Could you check a few things on this model? Use its own coordinates, in mm. A direction names the side the tool comes from. Coordinates: 2 decimals unless noted, no trailing zeros. One line per question, with ' | ' between items.
```python
from build123d import *

# Parameters (mm, degrees)
BOSS_EXTRUDE1_DEPTH = 6
SKETCH2_R           = 5
CUT_EXTRUDE1_DEPTH  = 6
SKETCH11_R          = 4.999999998
CUT_EXTRUDE2_DEPTH  = 10
SKETCH12_R          = 5
SKETCH12_R_2        = 2.5
CUT_EXTRUDE3_DEPTH  = 10
CUT_EXTRUDE4_DEPTH  = 10
CUT_EXTRUDE5_DEPTH  = 10
BOSS_EXTRUDE2_START = -6
SKETCH14_R          = 2.5
BOSS_EXTRUDE2_DEPTH = 6
SKETCH14_3_R        = 2.5
CUT_EXTRUDE6_DEPTH  = 6
SKETCH11_4_R        = 4.999999998
BOSS_EXTRUDE3_DEPTH = 6


with BuildPart() as part:
    # Sketch1 → Boss-Extrude1 (new body)
    with BuildSketch(Plane.XY):
        Polygon((-82.808015356, -91.768584182), (61.688025962, -107.113154668), (120.9333121, 25.569013955), (13.052871288, 122.915674351), (-112.866193993, 50.397050544), align=None)
    extrude(amount=BOSS_EXTRUDE1_DEPTH)

    # Sketch2 → Cut-Extrude1 (cut)
    with BuildSketch(Plane.XY.offset(6)):
        Circle(SKETCH2_R)
    extrude(amount=-CUT_EXTRUDE1_DEPTH, mode=Mode.SUBTRACT)

    # Sketch11 → Cut-Extrude2 (cut)
    with BuildSketch(Plane.XY.offset(6)):
        with Locations((-6.54719671, -61.653339044)):
            Circle(SKETCH11_R)
        with Locations((-4.672797652, -44.002584721)):
            Circle(SKETCH11_R)
        with Locations((-2.798398593, -26.351830398)):
            Circle(SKETCH11_R)
        with Locations((-8.975995491, -84.524739011)):
            Circle(SKETCH11_R)
    cut_extrude2 = extrude(amount=-CUT_EXTRUDE2_DEPTH, mode=Mode.SUBTRACT)

    # Sketch12 → Cut-Extrude3 (cut)
    with BuildSketch(Plane.XY.offset(6)):
        with Locations((48.851207931, -21.813057641)):
            Circle(SKETCH12_R)
        with Locations((25.110433983, -11.212319348)):
            Circle(SKETCH12_R)
        with Locations((84.822429951, -20.352343286)):
            Circle(SKETCH12_R_2)
        with Locations((72.591981879, -32.413795933)):
            Circle(SKETCH12_R)
    cut_extrude3 = extrude(amount=-CUT_EXTRUDE3_DEPTH, mode=Mode.SUBTRACT)

    # Sketch11_3 → Cut-Extrude4 (cut)
    with BuildSketch(Plane.XY.offset(6)):
        Polygon((8.29449613, -101.443097727), (8.875295839, -95.973849909), (23.791426251, -97.557849113), (23.210626543, -103.027096932), align=None)
        Polygon((-29.414485521, -97.438641123), (-28.833685813, -91.969393305), (-43.749816225, -90.3853941), (-44.330615934, -95.854641919), align=None)
    cut_extrude4 = extrude(amount=-CUT_EXTRUDE4_DEPTH, mode=Mode.SUBTRACT)

    # Mirror3: Cut-Extrude2 across plane
    add(cut_extrude2.mirror(Plane(origin=(0, 0, 0), x_dir=(0, 0, 1), z_dir=(-0.4077207035645653, -0.9131066903077734, 0))), mode=Mode.SUBTRACT)

    # Mirror4: Cut-Extrude3 across plane
    add(cut_extrude3.mirror(Plane(origin=(0, 0, 0), x_dir=(0, 0, 1), z_dir=(0.742423441529948, -0.6699309169360882, 0))), mode=Mode.SUBTRACT)

    # Mirror5: Cut-Extrude2 across plane
    add(cut_extrude2.mirror(Plane(origin=(0, 0, 0), x_dir=(0, 0, 1), z_dir=(0.742423441529948, -0.6699309169360882, 0))), mode=Mode.SUBTRACT)

    # Mirror6: Cut-Extrude4 across plane
    add(cut_extrude4.mirror(Plane(origin=(0, 0, 0), x_dir=(0, 0, 1), z_dir=(-0.4077207035645653, -0.9131066903077734, 0))), mode=Mode.SUBTRACT)

    # Mirror7: Cut-Extrude4 across plane
    add(cut_extrude4.mirror(Plane(origin=(0, 0, 0), x_dir=(0, 0, 1), z_dir=(0.742423441529948, -0.6699309169360882, 0))), mode=Mode.SUBTRACT)

    # Sketch13 → Cut-Extrude5 (cut)
    with BuildSketch(Plane.XY.offset(6)):
        Polygon((79.910592339, -66.30299436), (102.710745723, -15.241146353), (97.688658926, -12.998682483), (74.888505542, -64.060530491), align=None)
    cut_extrude5 = extrude(amount=-CUT_EXTRUDE5_DEPTH, mode=Mode.SUBTRACT)

    # Mirror8: Cut-Extrude5 across plane
    add(cut_extrude5.mirror(Plane(origin=(0, 0, 0), x_dir=(0, 0, 1), z_dir=(0.742423441529948, -0.6699309169360882, 0))), mode=Mode.SUBTRACT)

    # Sketch14 → Boss-Extrude2 (add)
    with BuildSketch(Plane(origin=(0, 0, 0), x_dir=(-1, 0, 0), z_dir=(0, 0, -1)).offset(BOSS_EXTRUDE2_START)):
        with Locations((-84.822429951, -20.352343286)):
            Circle(SKETCH14_R)
    extrude(amount=BOSS_EXTRUDE2_DEPTH)

    # Sketch14_3 → Cut-Extrude6 (cut)
    with BuildSketch(Plane(origin=(0, 0, 0), x_dir=(-1, 0, 0), z_dir=(0, 0, -1))):
        with Locations(Location((-71.775367437, -49.571757376, 0), (0, 0, 180))):
            Circle(SKETCH14_3_R)
    extrude(amount=-CUT_EXTRUDE6_DEPTH, mode=Mode.SUBTRACT)

    # Sketch11_4 → Boss-Extrude3 (add)
    with BuildSketch(Plane.XY.offset(6)):
        Polygon((8.875295839, -95.973849909), (8.29449613, -101.443097727), (23.210626543, -103.027096932), (23.791426251, -97.557849113), align=None)
        Polygon((-44.330615934, -95.854641919), (-29.414485521, -97.438641123), (-28.833685813, -91.969393305), (-43.749816225, -90.3853941), align=None)
        with Locations((-6.54719671, -61.653339044)):
            Circle(SKETCH11_4_R)
        with Locations((-4.672797652, -44.002584721)):
            Circle(SKETCH11_4_R)
        with Locations((-2.798398593, -26.351830398)):
            Circle(SKETCH11_4_R)
        with Locations((-8.975995491, -84.524739011)):
            Circle(SKETCH11_4_R)
    extrude(amount=-BOSS_EXTRUDE3_DEPTH)

    # Mirror9: Cut-Extrude3, Cut-Extrude5 across plane
    add(cut_extrude3.mirror(Plane(origin=(0, 0, 0), x_dir=(0, 0, 1), z_dir=(0.8665636244747431, 0.4990666135268884, 0))), mode=Mode.SUBTRACT)
    add(cut_extrude5.mirror(Plane(origin=(0, 0, 0), x_dir=(0, 0, 1), z_dir=(0.8665636244747431, 0.4990666135268884, 0))), mode=Mode.SUBTRACT)


solid = part.part
```
Q1. For faces 1 (the face through (43.742, 87.815, 3.042)), 2 (the face through (-88.084, -53.335, 3.042)), 3 (the face through (70.672, -86.994, 2.958)), 4 (the face through (-38.078, -93.792, 3.042)), which set-ups out of +Z, -Z, +X, -X, +Y, -Y let a thin tool reach every point of the face, with its end or its side?
Values follow:
face 1: +Z, -Z | face 2: +Z, -Z, -X | face 3: +Z, -Z, +X, -Y | face 4: +Z, -Z, -Y
Q2. Imagine slicing it at A-A on z = 5. Give the number of separate pieces and of enclosed holes in the cut face, plus the area to 3 significant figures.
Values follow:
separate pieces: 1 | enclosed holes: 21 | area: 33,600 mm2
Q3. Please list where these lines run through material, in increasing order: L1, parallel to X at y = 84, z = 4.25; L2, parallel to Y at x = 75, z = 3.25; L3, parallel to X at y = -7.5, z = 4.75. Write a range as [from, to].
Values follow:
L1: x = [-43.5, -30.76], [-27.1, 47.97], [50.26, 56.18] | L2: y = [-77.3, -64.11], [-63.81, -36.8], [-28.03, 67.02] | L3: x = [-100.62, -48.01], [-38.57, -30.5], [-21.35, 21.76], [28.46, 106.17]
Q4. For pin 1 (2 mm diameter, centred on x = 53.5, z = 4, fed in from -Y); pin 2 (8 mm diameter, centred on x = 48.85, y = -21.81, fed in from +Z); pin 3 (2 mm diameter, centred on x = -29, z = 3, fed in from -Y); pin 4 (2 mm diameter, centred on y = 19.5, z = 4, fed in from +X), each with a flat end and sliding along its axis, tell me the tip position at first contact or that it passes through.
Values follow:
pin 1: stops at y = -106.35 | pin 2: passes through | pin 3: stops at y = -92.06 | pin 4: stops at x = 118.67
Q5. We'd pull the mould along X, two halves only. Please class faces 5 (the face through (-99.106, -1.574, 3.042)), 6 (the face through (2, 10, 0)), 7 (the face through (100.235, -14.136, 3.042)): released by +X, released by -X, zero draft, split by the parting line, or undercut.
Values follow:
face 5: released by -X | face 6: zero draft | face 7: undercut
